Verification items for the finished model (mm, model axes). A direction names the side the tool comes from. Coordinates: 2 decimals unless noted, no trailing zeros. Write each loop counter-clockwise with the first axis right and the second up, starting at its lowest first coordinate (ties: lowest second). Pieces come first, ordered by that corner, then holes. Notation, with made-up numbers: (-22.75, 41) - (-11.75, 41) arc R12 cw to (-11.75, 62) - close; hole circle Ø9 at (-11.5, -23.75). An arc over 180 degrees is marked (long way). Use one line per item in the form item = value. Start each with the question number.
(1) Sectioned sample at B-B (x = 519). Record the cut outline in (y, z), and give its area (3 significant figures).
(2) Mould release check, pull along Y, two halves, no side actions. Record for faces 3 (the flat face through (526.293, 520.225, 29.58)), 4 (the flat face through (700, -4, 30)), 5 (the flat face through (740, -4, 30)), 6 (the flat face through (4.1, 700, 22.9)): released by +Y, released by -Y, zero draft, split by the parting line, or undercut.
(3) Tool access check on faces 1 (the flat face through (497.85, 492.1, 29.58)), 2 (the flat face through (4.3, 740, 22.9)). Record the directions out of +Z, -Z, +X, -X, +Y, -Y that give a thin tool (end or side, any length) a straight path to the whole face; none if there is none.
(4) Gauge pin test, flat ends, axial feed: pin 1 Ø14 at (y, z) = (-45, 15) entering from -X; pin 2 Ø11 at (y, z) = (45, 45) entering from -X; pin 3 Ø8 at (y, z) = (-515.5, 29) entering from -X; pin 4 Ø8 at (x, z) = (-449, 35) entering from -Y. Record the tip position at first contact, or that the pin passes through.
(5) Material ranges on line 1 (Y direction, x = -28, z = 20); line 2 (Y direction, x = 726, z = 15), recorded low to high. Write a range as [from, to].
(6) Sectioned sample at A-A (x = -88). Record the cut outline in (y, z).
from build123d import *

# Parameters (mm, degrees)
BOSS_EXTRUDE1_DEPTH = 60
SKETCH4_R           = 8
SKETCH4_R_2         = 6
CUT_EXTRUDE1_DEPTH  = 1968
SKETCH6_R           = 6
CUT_EXTRUDE2_DEPTH  = 1968


with BuildPart() as part:
    # Sketch2 → Boss-Extrude1 (new body)
    with BuildSketch(Plane.XY):
        Polygon((740, 306.518036156), (306.518036156, 740), (-306.518036156, 740), (-740, 306.518036156), (-740, -306.518036156), (-306.518036156, -740), (306.518036156, -740), (740, -306.518036156), align=None)
        Polygon((700, -289.949493661), (700, 289.949493661), (289.949493661, 700), (-289.949493661, 700), (-700, 289.949493661), (-700, -289.949493661), (-289.949493661, -700), (289.949493661, -700), align=None, mode=Mode.SUBTRACT)
    extrude(amount=BOSS_EXTRUDE1_DEPTH)

    # Sketch4 → Cut-Extrude1 (cut)
    with BuildSketch(Plane.XZ.offset(740)):
        with Locations(Location((0, 30, 0), (0, 0, 270))):
            Circle(SKETCH4_R)
        with Locations(Location((-45, 30, 0), (0, 0, 270))):
            Circle(SKETCH4_R_2)
        with Locations(Location((45, 30, 0), (0, 0, 270))):
            Circle(SKETCH4_R_2)
    extrude(amount=-CUT_EXTRUDE1_DEPTH, mode=Mode.SUBTRACT)

    # Sketch6 → Cut-Extrude2 (cut)
    with BuildSketch(Plane(origin=(740, 0, 0), x_dir=(0, 0, -1), z_dir=(1, 0, 0))):
        with Locations((-15, 45)):
            Circle(SKETCH6_R)
        with Locations((-15, -45)):
            Circle(SKETCH6_R)
        with Locations((-45, 45)):
            Circle(SKETCH6_R)
        with Locations((-45, -45)):
            Circle(SKETCH6_R)
    extrude(amount=-CUT_EXTRUDE2_DEPTH, mode=Mode.SUBTRACT)


solid = part.part
Answers below:
q1.outline = (-527.52, 0) - (-470.95, 0) - (-470.95, 60) - (-527.52, 60) - close; (470.95, 0) - (527.52, 0) - (527.52, 60) - (470.95, 60) - close
q1.area = 6,790 mm2
q2.face_3 = released by +Y
q2.face_4 = undercut
q2.face_5 = zero draft
q2.face_6 = undercut
q3.face_1 = +Z, -Z
q3.face_2 = +Z, -Z, +X, -X, +Y
q4.pin_1 = -740
q4.pin_2 = through
q4.pin_3 = -535.02
q4.pin_4 = -601.52
q5.line_1 = [-740, -700], [700, 740]
q5.line_2 = [-320.52, -51], [-39, 39], [51, 320.52]
q6.outline = (-740, 0) - (-700, 0) - (-700, 60) - (-740, 60) - close; (700, 0) - (740, 0) - (740, 60) - (700, 60) - close
